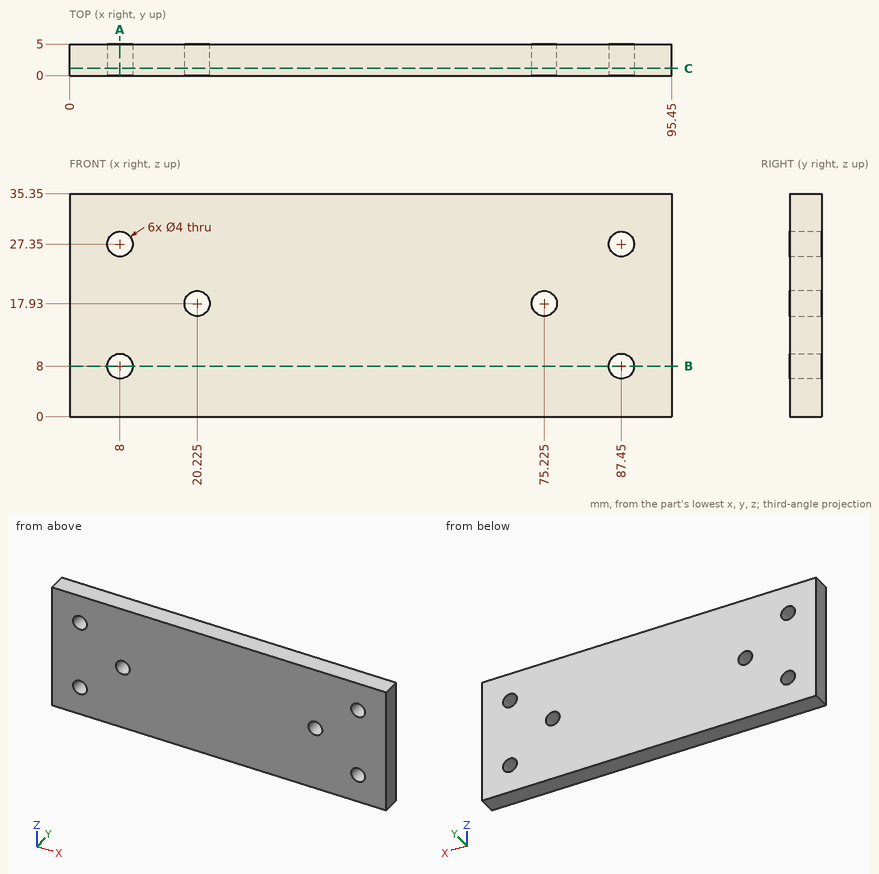
Study the drawing (mm; zero at the part's minimum x, y, z) and answer. Coordinates: 2 decimals unless noted, no trailing zeros. Loops run counter-clockwise (first coordinate to the right, second up) from the corner with the lowest first, then second, coordinate; pieces in that order, holes last. Notation, with made-up numbers: (27, 89.25) -> (75, 89.25) arc R37 cw to (75, 125.25) -> close; hole circle Ø7 at (28, -1.5). An arc over 180 degrees is marked (long way). Answer in a Markdown table with one row per item. Add a question column.
1. The part is cut by section B-B, the plane z = 8. Write down the section's boundary in (x, y), then the cut area to 3 significant figures.
2. The part is cut by section A-A, the plane x = 8. Write down the section's boundary in (y, z), then the cut area to 3 significant figures.
3. Consider line 1 (X direction, y = 1.65, z = 8); line 2 (X direction, y = 1.5, z = 26.5); line 3 (Z direction, x = 88, y = 0.3). Determine where each line is inside the solid, lowest interval first. Write a range as [from, to].
4. The part is cut by section C-C, the plane y = 1.15. Count the separate pieces of the cut face and the enclosed holes in it, then the cut area to 3 significant figures.
Answer below:
| question | item | result |
|---|---|---|
| 1 | outline | (0, 0) -> (6, 0) -> (6, 5) -> (0, 5) -> close; (10, 0) -> (85.45, 0) -> (85.45, 5) -> (10, 5) -> close; (89.45, 0) -> (95.45, 0) -> (95.45, 5) -> (89.45, 5) -> close |
| 1 | area | 437 mm2 |
| 2 | outline | (0, 0) -> (5, 0) -> (5, 6) -> (0, 6) -> close; (0, 10) -> (5, 10) -> (5, 25.35) -> (0, 25.35) -> close; (0, 29.35) -> (5, 29.35) -> (5, 35.35) -> (0, 35.35) -> close |
| 2 | area | 137 mm2 |
| 3 | line 1 | [0, 6], [10, 85.45], [89.45, 95.45] |
| 3 | line 2 | [0, 6.19], [9.81, 85.64], [89.26, 95.45] |
| 3 | line 3 | [0, 6.08], [9.92, 25.43], [29.27, 35.35] |
| 4 | separate pieces | 1 |
| 4 | enclosed holes | 6 |
| 4 | area | 3,300 mm2 |
